Input: dimensioned drawing with shaded views. Units: mm. Origin: part minimum x, y, z. A direction names the side the tool comes from. Round coordinates to 2 decimals unless told otherwise and drop trailing zeros. Loops run counter-clockwise (first coordinate to the right, second up) from the corner with the lowest first, then second, coordinate; pieces in that order, holes last. Notation, with made-up numbers: (-16.75, 39) - (-4.75, 39) arc R32 cw to (-4.75, 75) - close; hole circle Ø9 at (-39, 83.25). An arc over 180 degrees is marked (long way). Answer as a JSON object with one key per item and string values. Group by question number.
Item 1: Section B-B (y = 9.5). Return the cut outline in (x, z) (1 decimal).
Item 2: Section C-C (x = 30.5). Return the cut outline in (y, z) (1 decimal), plus the area to 3 significant figures.
Item 3: Section D-D (z = 20). Return the cut outline in (x, y).
Item 4: Draft query along X for the marked faces 4, 5 and 6. Return one class per face: released by +X, released by -X, zero draft, split by the parting line, or undercut.
Item 5: Reachability of the marked faces 1, 2 and 3 from +Z, -Z, +X, -X, +Y, -Y: full face, straight path, thin tool, end or side. Return the list, or none.
Item 6: First-contact query: pin 1 (10 mm diameter, centred on x = 87, y = 91.5, fed in from +Z); pin 2 (4 mm diameter, centred on y = 131.37, z = 4.13, fed in from -X); pin 3 (4 mm diameter, centred on x = 41, y = 71.5, fed in from -Z); pin 4 (5 mm diameter, centred on x = 39, z = 60.5, fed in from +Y). Flat tips, straight axial feed; report the tip coordinate or a pass-through.
Item 7: Section A-A (z = 27). Return the cut outline in (x, y).
Item 8: Line query: line 1 (Y direction, x = 64, z = 58.5); line 2 (Z direction, x = 63.5, y = 68.5); line 3 (Y direction, x = 41, z = 43). Output: solid intervals per line, ascending.
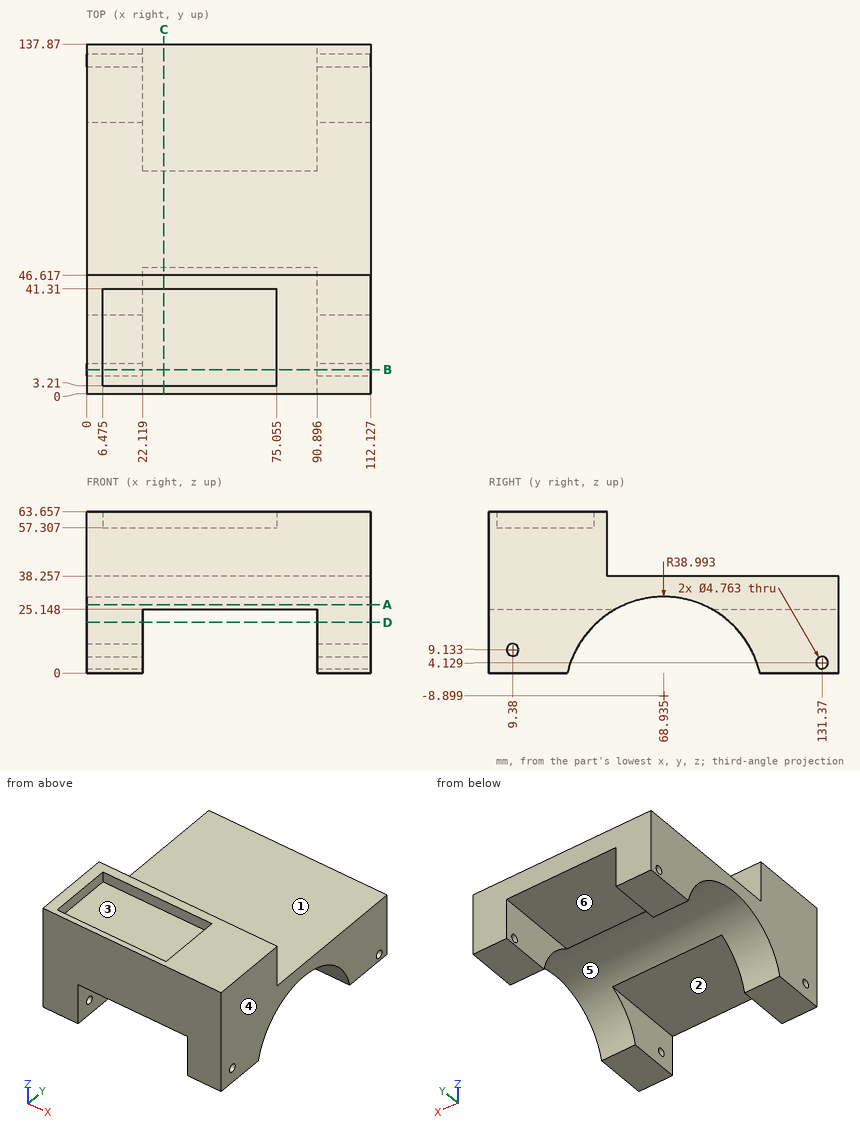
Values:
{
 "1": {"outline": "(0, 0) - (22.1, 0) - (22.1, 6.8) - (0, 6.8) - close; (0, 11.5) - (22.1, 11.5) - (22.1, 25.1) - (90.9, 25.1) - (90.9, 11.5) - (112.1, 11.5) - (112.1, 63.7) - (75.1, 63.7) - (75.1, 57.3) - (6.5, 57.3) - (6.5, 63.7) - (0, 63.7) - close; (90.9, 0) - (112.1, 0) - (112.1, 6.8) - (90.9, 6.8) - close"},
 "2": {"outline": "(0, 25.1) - (49.9, 25.1) arc R39 cw to (87.9, 25.1) - (137.9, 25.1) - (137.9, 38.3) - (46.6, 38.3) - (46.6, 63.7) - (41.3, 63.7) - (41.3, 57.3) - (3.2, 57.3) - (3.2, 63.7) - (0, 63.7) - close", "area": "2,620 mm^2"},
 "3": {"outline": "(0, 0) - (22.12, 0) - (22.12, 42.76) - (0, 42.76) - close; (0, 95.11) - (22.12, 95.11) - (22.12, 137.87) - (0, 137.87) - close; (90.9, 0) - (112.13, 0) - (112.13, 42.76) - (90.9, 42.76) - close; (90.9, 95.11) - (112.13, 95.11) - (112.13, 137.87) - (90.9, 137.87) - close"},
 "4": {"face 4": "released by +X", "face 5": "zero draft", "face 6": "undercut"},
 "5": {"face 1": "+Z, +X, -X, +Y", "face 2": "-Z, +Y, -Y", "face 3": "+Z"},
 "6": {"pin 1": "stops at z = 38.26", "pin 2": "passes through", "pin 3": "stops at z = 29.83", "pin 4": "stops at y = 46.62"},
 "7": {"outline": "(0, 0) - (112.13, 0) - (112.13, 53.71) - (0, 53.71) - close; (0, 84.16) - (112.13, 84.16) - (112.13, 137.87) - (0, 137.87) - close"},
 "8": {"line 1": "y = 0 to 3.21, 41.31 to 46.62", "line 2": "z = 30.09 to 38.26", "line 3": "y = 0 to 46.62"}
}
